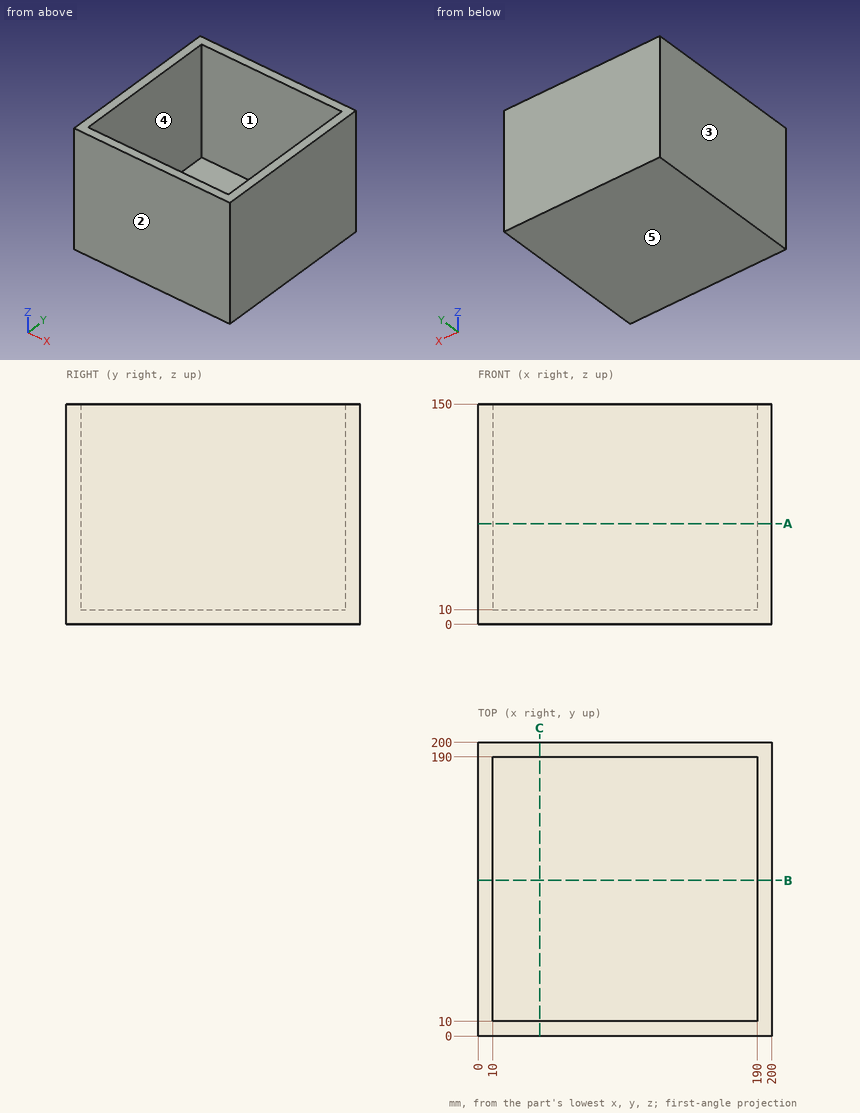
Print and shaded views of the part. All mm, measured from the part's lowest x, y and z. A direction names the side the tool comes from. Coordinates: 2 decimals unless noted, no trailing zeros. Loops run counter-clockwise (first coordinate to the right, second up) from the corner with the lowest first, then second, coordinate; pieces in that order, holes last. Notation, with made-up numbers: M -4.5,-39 L 7.5,-39 A15 ccw 7.5,-26 Z; hole C 57,68.5 d10. An arc over 180 degrees is marked long. Use a Markdown table: item, result. Add a question column.
Q1. Probe L1, parallel to X at y = 66, z = 66.5; L2, parallel to Z at x = 132.5, y = 40. List the from-to ranges inside material, lowest first.
Q2. Cut at B-B (y = 106). Write the cut outline in (x, z).
Q3. Pin check, flat tips, straight feed: P1, Ø2, axis at x = 141, y = 156, coming from the -Z side; P2, Ø2, axis at x = 161, y = 97.5, coming from the +Z side. Stop position of each tip, or through.
Q4. Mould opens along X. For the marked faces 3, 4 and 5 say: +X half, -X half, draft (parallel to the pull), parting line (faces both ways), or undercut.
Q5. Which spindle directions (+Z, -Z, +X, -X, +Y, -Y) get a long thin tool onto all of the face, cutting with end or side? Do the marked faces 1 and 2. Say none if no direction does.
Q6. Cut at A-A (z = 68.5). Write the cut outline in (x, y), and give its area (3 significant figures).
Worked out:
| question | item | result |
|---|---|---|
| 1 | L1 | x = 0 to 10, 190 to 200 |
| 1 | L2 | z = 0 to 10 |
| 2 | outline | M 0,0 L 200,0 L 200,150 L 190,150 L 190,10 L 10,10 L 10,150 L 0,150 Z |
| 3 | P1 | stops at z = 0 |
| 3 | P2 | stops at z = 10 |
| 4 | face 3 | -X half |
| 4 | face 4 | undercut |
| 4 | face 5 | draft |
| 5 | face 1 | +Z |
| 5 | face 2 | +Z, -Z, +X, -X, -Y |
| 6 | outline | M 0,0 L 200,0 L 200,200 L 0,200 Z; hole M 10,10 L 190,10 L 190,190 L 10,190 Z |
| 6 | area | 7,600 mm2 |
